Can you work these out from the model? Positions are in its coordinate system, mm. Round coordinates to 2 decimals unless told otherwise and drop trailing zeros. Order: outer loops, then holes, each group sorted by start corner. A loop starts at its lowest first (then second) coordinate and runs counter-clockwise, first axis right, second up. Notation, with made-up numbers: (5.5, 59) -> (58.5, 59) arc R26 ccw to (58.5, 77) -> close; hole circle Ø7 at (81, 67.25). An arc over 180 degrees is marked (long way). Use a Markdown table: item, result. Add a question column.
Q1. If we section it at A-A on z = 0.8: List the corners of the cut face in (x, y) for me (3 decimals), plus the area to 3 significant figures.
Q2. If we section it at C-C on x = 17: List the corners of the cut face in (y, z) for me.
Q3. If we section it at B-B on x = 0: List the corners of the cut face in (y, z) for me (3 decimals), plus the area to 3 significant figures.
Q4. I need wall thicknesses on line 1 along Y through (x, z) = (0, 0.6) (3 decimals); line 2 along X through (y, z) = (-19, 0.05); line 3 along Y through (x, z) = (16.5, 0.95). Which ranges of each line are inside material? Lowest first, please. Write a range as [from, to].
```python
from build123d import *

# Parameters (mm, degrees)
F0_R     = 6.475
F0_R_2   = 8.075
F1_DEPTH = 1


with BuildPart() as f1:
    # F0 (on Top) → F1 (new body)
    with BuildSketch(Plane.XY):
        with BuildLine():
            ThreePointArc((20.655149, 46.151557), (-0.075475, 40.918495), (-20.825263, 46.075046))
            ThreePointArc((-20.825263, 46.075046), (-26.653292, 45.968832), (-29.640847, 40.963663))
            ThreePointArc((-29.640847, 40.963663), (-35.474194, 20.393884), (-50.314792, 5.002316))
            ThreePointArc((-50.314792, 5.002316), (-53.136822, -0.098012), (-50.295996, -5.187895))
            ThreePointArc((-50.295996, -5.187895), (-35.398719, -20.524611), (-29.489529, -41.07273))
            ThreePointArc((-29.489529, -41.07273), (-26.48353, -46.066844), (-20.655149, -46.151557))
            ThreePointArc((-20.655149, -46.151557), (0.075475, -40.918495), (20.825263, -46.075046))
            ThreePointArc((20.825263, -46.075046), (26.653292, -45.968832), (29.640847, -40.963663))
            ThreePointArc((29.640847, -40.963663), (35.474194, -20.393884), (50.314792, -5.002316))
            ThreePointArc((50.314792, -5.002316), (53.136822, 0.098012), (50.295996, 5.187895))
            ThreePointArc((50.295996, 5.187895), (35.398719, 20.524611), (29.489529, 41.07273))
            ThreePointArc((29.489529, 41.07273), (26.48353, 46.066844), (20.655149, 46.151557))
        make_face()
        with Locations((-12.460044, -21.673655)):
            Circle(F0_R, mode=Mode.SUBTRACT)
        with Locations((-24.999957, -0.046113)):
            Circle(F0_R, mode=Mode.SUBTRACT)
        with Locations((12.539914, -21.627542)):
            Circle(F0_R, mode=Mode.SUBTRACT)
        with Locations((-12.539914, 21.627542)):
            Circle(F0_R, mode=Mode.SUBTRACT)
        Circle(F0_R_2, mode=Mode.SUBTRACT)
        with Locations((24.999957, 0.046113)):
            Circle(F0_R, mode=Mode.SUBTRACT)
        with Locations((12.460044, 21.673655)):
            Circle(F0_R, mode=Mode.SUBTRACT)
    extrude(amount=F1_DEPTH)


solid = f1.part
```
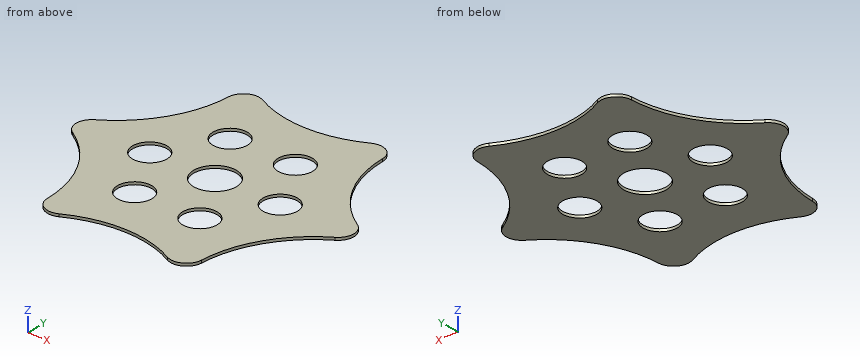
Answer below:
| question | item | result |
|---|---|---|
| 1 | outline | (-50.315, 5.002) arc R6 ccw to (-50.296, -5.188) arc R44 cw to (-29.49, -41.073) arc R6 ccw to (-20.655, -46.152) arc R44 cw to (20.825, -46.075) arc R6 ccw to (29.641, -40.964) arc R44 cw to (50.315, -5.002) arc R6 ccw to (50.296, 5.188) arc R44 cw to (29.49, 41.073) arc R6 ccw to (20.655, 46.152) arc R44 cw to (-20.825, 46.075) arc R6 ccw to (-29.641, 40.964) arc R44 cw to start; hole circle Ø12.95 at (-25, -0.046); hole circle Ø12.95 at (-12.54, 21.628); hole circle Ø12.95 at (-12.46, -21.674); hole circle Ø16.15 at (0, 0); hole circle Ø12.95 at (12.46, 21.674); hole circle Ø12.95 at (12.54, -21.628); hole circle Ø12.95 at (25, 0.046) |
| 1 | area | 5,530 mm² |
| 2 | outline | (-44.27, 0) -> (-26.32, 0) -> (-26.32, 1) -> (-44.27, 1) -> close; (-16.93, 0) -> (17.06, 0) -> (17.06, 1) -> (-16.93, 1) -> close; (26.29, 0) -> (44.4, 0) -> (44.4, 1) -> (26.29, 1) -> close |
| 3 | outline | (-40.919, 0) -> (-8.075, 0) -> (-8.075, 1) -> (-40.919, 1) -> close; (8.075, 0) -> (40.919, 0) -> (40.919, 1) -> (8.075, 1) -> close |
| 3 | area | 65.7 mm² |
| 4 | line 1 | [-40.919, -8.075], [8.075, 40.919] |
| 4 | line 2 | [-36.32, -18.36], [-6.56, 6.62], [18.46, 36.31] |
| 4 | line 3 | [-44.07, -26.75], [-16.5, 16.61], [26.73, 44.19] |
